```python
from build123d import *

# Parameters (mm, degrees)
SKETCH2_W                 = 75
SKETCH2_H                 = 75
BOSS_EXTRUDE1_DEPTH       = 4.7625
M4X0_7_TAPPED_HOLE1_D     = 3.3
M4X0_7_TAPPED_HOLE1_DEPTH = 15
M4X0_7_TAPPED_HOLE1_TIP   = 0.991420021
SKETCH6_R                 = 29
CUT_EXTRUDE1_DEPTH        = 54.881588924
M4_CLEARANCE_HOLE1_D      = 4.5
FILLET1_R                 = 37.5
M2X0_4_TAPPED_HOLE1_D     = 1.6


with BuildPart() as part:
    # Sketch2 → Boss-Extrude1 (new, symmetric)
    with BuildSketch(Plane.XY):
        Rectangle(SKETCH2_W, SKETCH2_H)
    extrude(amount=BOSS_EXTRUDE1_DEPTH, both=True)

    # M4x0.7 Tapped Hole1
    with Locations(Plane(origin=(0, -37.5, 0), x_dir=(-1, 0, 0), z_dir=(0, -1, 0))):
        with Locations((-32.5, 0), (-22.5, 0), (22.5, 0), (32.5, 0)):
            Hole(M4X0_7_TAPPED_HOLE1_D / 2, depth=M4X0_7_TAPPED_HOLE1_DEPTH)
            with Locations((0, 0, -(M4X0_7_TAPPED_HOLE1_DEPTH + M4X0_7_TAPPED_HOLE1_TIP / 2))):  # 118° drill point
                Cone(0, M4X0_7_TAPPED_HOLE1_D / 2, M4X0_7_TAPPED_HOLE1_TIP, mode=Mode.SUBTRACT)

    # Sketch6 → Cut-Extrude1 (cut, through all)
    with BuildSketch(Plane.XY.offset(4.7625)):
        Circle(SKETCH6_R)
    extrude(amount=-CUT_EXTRUDE1_DEPTH, mode=Mode.SUBTRACT)

    # M4 Clearance Hole1 (through all)
    with Locations(Plane(origin=(0, 0, -4.7625), x_dir=(-1, 0, 0), z_dir=(0, 0, -1))):
        with Locations((0, 32.5), (28.145825623, 16.25), (-28.145825623, 16.25), (-28.145825623, -16.25), (0, -32.5), (28.145825623, -16.25)):
            Hole(M4_CLEARANCE_HOLE1_D / 2)

    # Fillet1
    fillet1_edges = [part.edges().sort_by_distance(p)[0] for p in [
        (-37.5, 37.5, 0),
        (37.5, 37.5, 0),
    ]]
    fillet(fillet1_edges, radius=FILLET1_R - 0.0001)  # a hair under: the kernel refuses the full size

    # M2x0.4 Tapped Hole1 (through all)
    with Locations(Plane.XY.offset(4.7625)):
        with Locations((27.5, -30.38125)):
            Hole(M2X0_4_TAPPED_HOLE1_D / 2)


solid = part.part
```
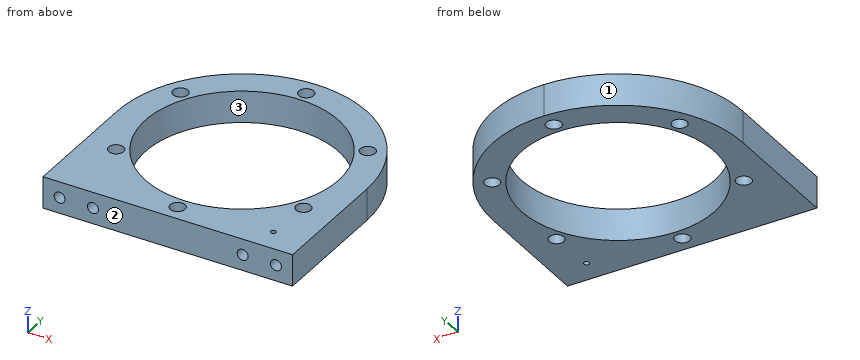
For this review, take the finished solid that the model builds, in its own axes (mm). Face numbers are marked on the shaded views. Give positions to 0.01 mm unless a question says otherwise; leave off trailing zeros. Write each loop counter-clockwise with the first axis right and the second up, starting at its lowest first coordinate (ties: lowest second). Pieces come first, ordered by that corner, then holes.
Item 1: Take a section at A-A (y = -32.5). Give the boundary of the cut face in (x, z).
Item 2: Wall thickness on probe 1 along Y at (x, z) = (0, -2); probe 2 along Y at (x, z) = (-29.5, 0.75); probe 3 along Y at (x, z) = (-12.5, 3.5): over which ranges is each line inside the solid? List them lowest first.
Item 3: Take a section at B-B (x = 14). Give the boundary of the cut face in (y, z).
Item 4: Take a section at D-D (z = -3.5). Give the number of separate pieces and of enclosed holes in the cut face, and give its area (3 significant figures).
Item 5: Insertion check: P1, Ø4.5, axis at x = 22.5, z = 0, coming from the +Y side; P2, Ø3, axis at x = 32.5, z = 0, coming from the +Y side; P3, Ø1.4, axis at x = 27.5, y = -30.38, coming from the +Z side; P4, Ø4, axis at x = -22.5, z = 0, coming from the +Y side. Each pin has a flat end and moves straight along its axis. Give the tip position at first contact, or say it passes through.
Item 6: The part is to be moulded in two halves that separate along X. For the marked faces 1, 2 and 3, say which applies: +X half, -X half, draft (parallel to the pull), parting line (faces both ways), or undercut.
Item 7: Take a section at C-C (y = -16.25). Give the boundary of the cut face in (x, z), and give its area (3 significant figures).
Established:
1. outline: (-37.5, -4.76) - (-2.25, -4.76) - (-2.25, 4.76) - (-37.5, 4.76) - close; (2.25, -4.76) - (37.5, -4.76) - (37.5, 4.76) - (2.25, 4.76) - close; hole circle Ø3.3 at (-32.5, 0); hole circle Ø3.3 at (-22.5, 0); hole circle Ø3.3 at (22.5, 0); hole circle Ø3.3 at (32.5, 0)
2. probe 1: y = -37.5 to -34.75, -30.25 to -29, 29 to 30.25, 34.75 to 37.5
2. probe 2: y = -37.5 to -18.05, -14.45 to 14.45, 18.05 to 23.15
2. probe 3: y = -37.5 to -26.17, 26.17 to 35.36
3. outline: (-37.5, -4.76) - (-25.4, -4.76) - (-25.4, 4.76) - (-37.5, 4.76) - close; (25.4, -4.76) - (34.79, -4.76) - (34.79, 4.76) - (25.4, 4.76) - close
4. separate pieces: 1
4. enclosed holes: 8
4. area: 2,280 mm2
5. P1: stops at y = 31.56
5. P2: stops at y = 21.1
5. P3: passes through
5. P4: stops at y = 31.4
6. face 1: -X half
6. face 2: draft
6. face 3: undercut
7. outline: (-37.5, -4.76) - (-30.4, -4.76) - (-30.4, 4.76) - (-37.5, 4.76) - close; (-25.9, -4.76) - (-24.02, -4.76) - (-24.02, 4.76) - (-25.9, 4.76) - close; (24.02, -4.76) - (25.9, -4.76) - (25.9, 4.76) - (24.02, 4.76) - close; (30.4, -4.76) - (37.5, -4.76) - (37.5, 4.76) - (30.4, 4.76) - close
7. area: 171 mm2
